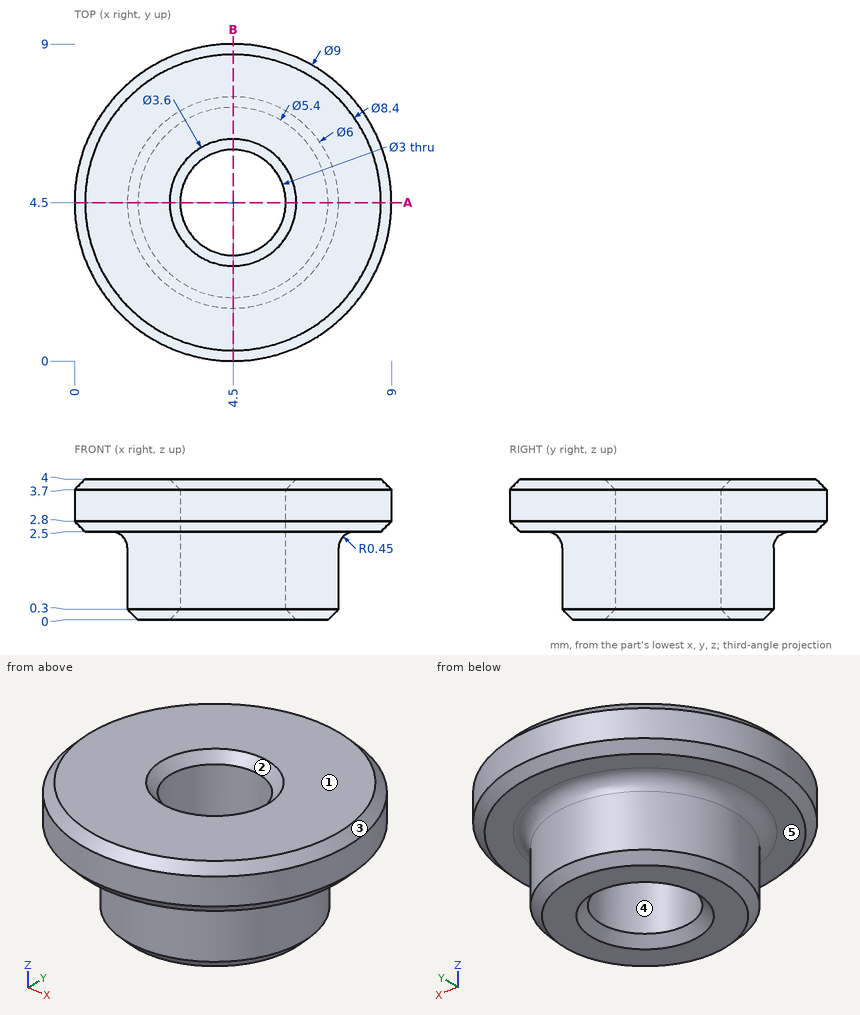
The drawing under review shows one solid part. Ordinate dimensions are in mm from its lowest x, y, z. A direction names the side the tool comes from. Round coordinates to 2 decimals unless told otherwise and drop trailing zeros. Order: outer loops, then holes, each group sorted by start corner. A loop starts at its lowest first (then second) coordinate and runs counter-clockwise, first axis right, second up. Notation, with made-up numbers: (49, -21) - (81, -21) arc R18 ccw to (81, 7) - close; hole circle Ø4 at (23, -7). An arc over 180 degrees is marked (long way). Return JSON: item names as keys, results as strings.
Q1. Machinability: for the marked faces 4 and 5, which of the approach directions +Z, -Z, +X, -X, +Y, -Y give a long, thin tool a straight path to every point of the face, cutting with its end or side? Answer none if there is none.
Computed values:
{"face 4": "+Z, -Z", "face 5": "-Z"}
Q2. Wall thickness on L1, parallel to Y at x = 4.5, z = 1.1; L2, parallel to X at y = 5.5, z = 3.35; L3, parallel to Z at x = 7.75, y = 5.5: over which ranges is each line inside the solid? List them lowest first. Write a range as [from, to].
Computed values:
{"L1": "y = [1.5, 3], [6, 7.5]", "L2": "x = [0.11, 3.38], [5.62, 8.89]", "L3": "z = [2.5, 4]"}
Q3. Consider section A-A on y = 4.5. Write out the cut boundary in (x, z), plus the area to 3 significant figures.
Computed values:
{"outline": "(0, 2.8) - (0.3, 2.5) - (1.05, 2.5) arc R0.45 cw to (1.5, 2.05) - (1.5, 0.3) - (1.8, 0) - (2.7, 0) - (3, 0.3) - (3, 3.7) - (2.7, 4) - (0.3, 4) - (0, 3.7) - close; (6, 0.3) - (6.3, 0) - (7.2, 0) - (7.5, 0.3) - (7.5, 2.05) arc R0.45 cw to (7.95, 2.5) - (8.7, 2.5) - (9, 2.8) - (9, 3.7) - (8.7, 4) - (6.3, 4) - (6, 3.7) - close", "area": "16.1 mm2"}
Q4. The part is to be moulded in two halves that separate along Y. For the marked faces 1, 2 and 3, say which applies: pulls with the +Y half, pulls with the -Y half, needs draft (parallel to the pull), parting line crosses it, or undercut.
Computed values:
{"face 1": "needs draft", "face 2": "undercut", "face 3": "parting line crosses it"}
Q5. For pin 1 Ø3 at (x, y) = (3.5, 5.5) entering from +Z; pin 2 Ø2 at (y, z) = (7, 0.5) entering from +X, all flat-tipped, find the tip position at first contact; note any pin that passes through.
Computed values:
{"pin 1": "stops at z = 4", "pin 2": "stops at x = 7.1"}
